Autodesk Inventor part; units mm, degrees
ref_plane "Work Plane1" through (-126.5, -50, 8) normal (0, 0, -1) x (0, 1, 0)
ref_plane "Work Plane2" through (-134.4075, -35.56, 12.6) normal (0, 0, -1) x (0, 1, 0)
ref_plane "YZ Plane" through (0, 0, 0) normal (1, 0, 0) x (0, 1, 0)
sketch "Sketch1" plane through (0, 0, 0) normal (0, 0, 1) x (1, 0, 0)
  line L0 (8, 57.5) -> (-137, 57.5)
  line L1 (-137, 57.5) -> (-137, -57.5)
  line L2 (-137, -57.5) -> (8, -57.5)
  line L3 (8, -57.5) -> (8, 57.5)
  line L4 (8, 0) -> (-137, 0) construction
  line L5 (-114.5, 49) -> (-74.5, 49)
  line L6 (-74.5, 49) -> (-74.5, -49)
  line L7 (-74.5, -49) -> (-114.5, -49)
  line L8 (-114.5, -49) -> (-114.5, 49)
  line L9 (-115.5, 50) -> (-73.5, 50)
  line L10 (-73.5, 50) -> (-73.5, -50)
  line L11 (-73.5, -50) -> (-115.5, -50)
  line L12 (-115.5, -50) -> (-115.5, 50)
  line L13 (2.5, 12.5) -> (-2.5, 12.5)
  line L14 (-2.5, 12.5) -> (-2.5, -12.5)
  line L15 (-2.5, -12.5) -> (2.5, -12.5)
  line L16 (2.5, -12.5) -> (2.5, 12.5)
  line L17 (3.25, -13.25) -> (-3.25, -13.25)
  line L18 (-3.25, -13.25) -> (-3.25, 13.25)
  line L19 (-3.25, 13.25) -> (3.25, 13.25)
  line L20 (3.25, 13.25) -> (3.25, -13.25)
  point P0 (0, 0)
  dimension "d0" = 115
  dimension "d1" = 145
  dimension "d2" = 8
  dimension "d3" = 1
  dimension "d4" = 0.75
extrude "Extrusion1" add sketch "Sketch1" along normal blind 3 contours L3 L2 L1 L0
sketch "Sketch2" plane through (0, 0, 3) normal (0, 0, 1) x (1, 0, 0)
  circle A0 centre (-67.5, -47) radius 1.7 construction
  circle A1 centre (-67.5, 47) radius 1.7 construction
  circle A2 centre (-121.5, 47) radius 1.7 construction
  circle A3 centre (-121.5, -47) radius 1.7 construction
  line L0 (-64.5, 50) -> (-124.5, 50) construction
  line L1 (-124.5, 50) -> (-124.5, -50) construction
  line L2 (-124.5, -50) -> (-64.5, -50) construction
  line L3 (-64.5, -50) -> (-64.5, 50) construction
  circle A4 centre (-67.5, 47) radius 2.7
  circle A5 centre (-121.5, 47) radius 2.7
  circle A6 centre (-67.5, -47) radius 2.7
  circle A7 centre (-121.5, -47) radius 2.7
  point P0 (0, 0)
  dimension "d7" = 1
ref_plane "Work Plane1" through (-126.5, -50, 8) normal (0, 0, -1) x (0, 1, 0)
extrude "Extrusion2" add sketch "Sketch2" along normal up to surface (5 mm away)
sketch "Sketch3" plane through (-121.5, 47, 8) normal (0, 0, 1) x (1, 0, 0)
  circle A0 centre (54, -94) radius 1.7 construction
  circle A1 centre (54, 0) radius 1.7 construction
  circle A2 centre (0, 0) radius 1.7 construction
  circle A3 centre (0, -94) radius 1.7 construction
  line L0 (57, 3) -> (-3, 3) construction
  line L1 (-3, 3) -> (-3, -97) construction
  line L2 (-3, -97) -> (57, -97) construction
  line L3 (57, -97) -> (57, 3) construction
  circle A4 centre (0, 0) radius 2.7 construction
  point P0 (121.5, -47)
hole "Hole1" at (-121.5, 47, 8) at (-121.5, -47, 8) at (-67.5, -47, 8) at (-67.5, 47, 8) direction (0, 0, -1) diameter 2.459 depth 5 tip angle 118
sketch "Sketch4" plane through (0, 0, 0) normal (0, 0, -1) x (-1, 0, 0)
  circle A0 centre (64, -30) radius 1.2 construction
  circle A1 centre (64, 30) radius 1.2 construction
  circle A2 centre (5, 30) radius 1.2 construction
  circle A3 centre (5, -30) radius 1.2 construction
  line L0 (66.5, 32.5) -> (2.5, 32.5) construction
  line L1 (2.5, 32.5) -> (2.5, -32.5) construction
  line L2 (2.5, -32.5) -> (66.5, -32.5) construction
  line L3 (66.5, -32.5) -> (66.5, 32.5) construction
  point P0 (0, 0)
hole "Hole2" at (-5, -30, 0) at (-5, 30, 0) at (-64, 30, 0) at (-64, -30, 0) direction (0, 0, 1) diameter 2.013 end through all
sketch "Sketch5" plane through (0, 0, 3) normal (0, 0, 1) x (1, 0, 0)
  circle A0 centre (-58.945, 32.258) radius 1.7 construction
  circle A1 centre (-127.525, -32.258) radius 1.7 construction
  circle A2 centre (-127.525, 32.258) radius 1.7 construction
  line L0 (-54.5, -35.56) -> (-54.5, 35.56) construction
  line L1 (-54.5, 35.56) -> (-131.97, 35.56) construction
  line L2 (-131.97, 35.56) -> (-131.97, -35.56) construction
  line L3 (-131.97, -35.56) -> (-54.5, -35.56) construction
  circle A3 centre (-127.525, 32.258) radius 2.7
  circle A4 centre (-58.945, 32.258) radius 2.7
  point P0 (0, 0)
  dimension "d24" = 1
ref_plane "Work Plane2" through (-134.4075, -35.56, 12.6) normal (0, 0, -1) x (0, 1, 0)
extrude "Extrusion3" add sketch "Sketch5" along normal up to surface (9.6 mm away)
sketch "Sketch6" plane through (-127.525, 32.258, 12.6) normal (0, 0, 1) x (1, 0, 0)
  circle A0 centre (0, 0) radius 2.7
  circle A1 centre (68.58, 0) radius 2.7
  point P0 (127.525, -32.258)
hole "Hole3" at (-127.525, 32.258, 12.6) at (-58.945, 32.258, 12.6) direction (0, 0, -1) diameter 2.459 depth 8.8 tip angle 118
ref_plane "Work Plane3" through (-137, 0, 0) normal (0, 1, 0) x (1, 0, 0)
mirror "Mirror1" about plane through (-137, 0, 0) normal (0, 1, 0) of "Extrusion3", "Hole3"
sketch "Sketch7" plane through (0, 0, 3) normal (0, 0, 1) x (1, 0, 0)
  circle A0 centre (-127.525, 32.258) radius 2.7 construction
  circle A1 centre (-58.945, 32.258) radius 2.7 construction
  circle A2 centre (-64, 30) radius 1.0065 construction
  circle A3 centre (-5, -30) radius 1.0065 construction
  circle A4 centre (-5, 30) radius 1.0065 construction
  circle A5 centre (-58.945, -32.258) radius 2.7 construction
  circle A6 centre (-64, -30) radius 1.0065 construction
  circle A7 centre (-67.5, -47) radius 2.7 construction
  circle A8 centre (-121.5, -47) radius 2.7 construction
  circle A9 centre (-121.5, 47) radius 2.7 construction
  circle A10 centre (-67.5, 47) radius 2.7 construction
  line L0 (-73.5, 50) -> (-73.5, -50) construction
  line L1 (-73.5, -50) -> (-115.5, -50) construction
  line L2 (-115.5, -50) -> (-115.5, 50) construction
  line L3 (-115.5, 50) -> (-73.5, 50) construction
  line L4 (-3.25, -13.25) -> (-3.25, 13.25) construction
  line L5 (-3.25, 13.25) -> (3.25, 13.25) construction
  line L6 (3.25, 13.25) -> (3.25, -13.25) construction
  line L7 (3.25, -13.25) -> (-3.25, -13.25) construction
  line L8 (8, 57.5) -> (-137, 57.5) construction
  line L9 (-137, 57.5) -> (-137, -57.5) construction
  line L10 (-137, -57.5) -> (8, -57.5) construction
  line L11 (8, -57.5) -> (8, 57.5) construction
  circle A11 centre (-127.525, -32.258) radius 2.7 construction
  line L12 (-137, 57.5) -> (-137, -57.5)
  line L13 (-137, -57.5) -> (8, -57.5)
  line L14 (-137, 57.5) -> (-132, 57.5)
  line L15 (-132, 57.5) -> (-132, -57.5)
  line L16 (-132, -57.5) -> (-137, -57.5)
  line L17 (-137, -57.5) -> (-137, 57.5)
  line L18 (8, 57.5) -> (-137, 57.5)
  line L19 (-115, 57.5) -> (-137, 57.5)
  line L20 (-137, 57.5) -> (-137, 53.5)
  line L21 (-137, 53.5) -> (-115, 53.5)
  line L22 (-115, 53.5) -> (-115, 57.5)
  line L23 (-137, 57.5) -> (-137, -57.5)
  line L24 (8, 0) -> (-137, 0)
  line L25 (8, -57.5) -> (-137, -57.5) construction
  line L26 (8, -57.5) -> (-137, -57.5)
  line L27 (-115, -53.5) -> (-115, -57.5)
  line L28 (8, 57.5) -> (-7, 57.5)
  line L29 (-7, 57.5) -> (-7, 52.5)
  line L30 (-7, 52.5) -> (8, 52.5)
  line L31 (8, 52.5) -> (8, 57.5)
  line L32 (8, -57.5) -> (-7, -57.5)
  line L33 (-7, -57.5) -> (-7, -52.5)
  line L34 (-7, -52.5) -> (8, -52.5)
  line L35 (8, -52.5) -> (8, -57.5)
  line L36 (-115, -53.5) -> (-137, -53.5)
  line L37 (-137, -53.5) -> (-137, -57.5)
  line L38 (-137, -57.5) -> (-115, -57.5)
  line L39 (-115, -57.5) -> (-115, -53.5)
  line L40 (8, 57.5) -> (3, 57.5)
  line L41 (3, 57.5) -> (3, 42.5)
  line L42 (3, 42.5) -> (8, 42.5)
  line L43 (8, 42.5) -> (8, 57.5)
  line L44 (8, -57.5) -> (8, 57.5)
  line L45 (8, -57.5) -> (3, -57.5)
  line L46 (3, -57.5) -> (3, -42.5)
  line L47 (3, -42.5) -> (8, -42.5)
  line L48 (8, -42.5) -> (8, -57.5)
  point P0 (0, 0)
  dimension "d34" = 5
  dimension "d35" = 22
  dimension "d36" = 4
  dimension "d37" = 15
  dimension "d38" = 5
extrude "Extrusion4" add sketch "Sketch7" along normal blind 30 contours L14 L15 L21 L12 | L21 L15 L24 L12 | L18 L22 L21 L15 | L24 L15 L36 L12 | L36 L15 L13 L12 | L18 L41 L30 L29 | L36 L27 L13 L15 | L18 L31 L30 L41 | L44 L34 L46 L47 | L42 L41 L30 L43 | L35 L13 L46 L34 | L33 L34 L46 L13
properties part number "Case"
Check sheet for the modelled part. Datum: model origin and axes. Units: mm. A direction names the side the tool comes from. Give positions to 0.01 mm unless a question says otherwise; leave off trailing zeros. Write each loop counter-clockwise with the first axis right and the second up, starting at its lowest first coordinate (ties: lowest second). Pieces come first, ordered by that corner, then holes. Notation, with made-up numbers: (77, 41) -> (122, 41) arc R25 ccw to (122, 73) -> close; hole circle Ø10 at (81.25, 77). An arc over 180 degrees is marked (long way). Use one line per item in the form item = value. Start each with the question number.
1. Go/stop test with flat-tipped pins: P1, Ø1.8, axis at x = -5, y = -30, coming from the -Z side; P2, Ø12, axis at x = -9.5, y = 22.5, coming from the +Z side; P3, Ø5, axis at y = 37, z = 17, coming from the +X side; P4, Ø4.5, axis at x = -59.5, y = 33.5, coming from the +Z side. Record where each tip stops, or that it passes through.
2. Section check B-B (x = -97). Record the cut outline in (y, z), and give its area (3 significant figures).
3. Access from +Z, -Z, +X, -X, +Y, -Y to the whole of each face (thin tool, end or side, straight path). Record for faces 3 (the cylindrical face through (-126.28, -29.86, 7.73)), 4 (the flat face through (-60, -31, 12.6)), 5 (the flat face through (3.25, 0, 1)).
4. Thickness scan on line 1 along X through (y, z) = (30, 1); line 2 along Y through (x, z) = (-5, 0.75); line 3 along Y through (x, z) = (-0.5, 10). Record the ranges inside material, lowest first. Write a range as from..to.
5. Section check C-C (z = 25.5). Record the cut outline in (x, y).
6. Mould release check, pull along X, two halves, no side actions. Record for faces 1 (the flat face through (3, -48, 18)), 2 (the flat face through (-75, 57.5, 1)): pulls with the +X half, pulls with the -X half, needs draft (parallel to the pull), parting line crosses it, or undercut.
7. Section check A-A (y = -39.5). Record the cut outline in (x, z), and give its area (3 significant figures).
Conclusion:
q1.P1 = through
q1.P2 = 3
q1.P3 = -132
q1.P4 = 12.6
q2.outline = (-57.5, 0) -> (-50, 0) -> (-50, 3) -> (-57.5, 3) -> close; (50, 0) -> (57.5, 0) -> (57.5, 3) -> (50, 3) -> close
q2.area = 45.0 mm²
q3.face_3 = +Z
q3.face_4 = +Z, +X, +Y, -Y
q3.face_5 = +Z, -Z
q4.line_1 = -137..-115.5, -73.5..-65.01, -62.99..-6.01, -3.99..8
q4.line_2 = -57.5..-31.01, -28.99..28.99, 31.01..57.5
q4.line_3 = -57.5..-52.5, 52.5..57.5
q5.outline = (-137, -57.5) -> (-115, -57.5) -> (-115, -53.5) -> (-132, -53.5) -> (-132, 53.5) -> (-115, 53.5) -> (-115, 57.5) -> (-137, 57.5) -> close; (-7, -57.5) -> (8, -57.5) -> (8, -42.5) -> (3, -42.5) -> (3, -52.5) -> (-7, -52.5) -> close; (-7, 52.5) -> (3, 52.5) -> (3, 42.5) -> (8, 42.5) -> (8, 57.5) -> (-7, 57.5) -> close
q6.face_1 = undercut
q6.face_2 = needs draft
q7.outline = (-137, 0) -> (-115.5, 0) -> (-115.5, 3) -> (-132, 3) -> (-132, 33) -> (-137, 33) -> close; (-73.5, 0) -> (8, 0) -> (8, 3) -> (-73.5, 3) -> close
q7.area = 459 mm²
